Input: dimensioned drawing with shaded views. Units: mm. Origin: part minimum x, y, z. A direction names the side the tool comes from. Coordinates: 2 decimals unless noted, no trailing zeros. Write each loop counter-clockwise with the first axis right and the second up, starting at its lowest first coordinate (ties: lowest second). Pieces come first, ordered by that corner, then holes. Notation, with made-up numbers: (74, 83) -> (82, 83) arc R24 ccw to (82, 122) -> close; hole circle Ø3 at (-26.5, 32.25). An arc over 180 degrees is marked (long way). One line per item, written item: value. Start each with the question number.
1. First-contact query: P1, Ø1.5, axis at y = 4.5, z = 11.5, coming from the -X side; P2, Ø2, axis at x = 3.5, y = 7.5, coming from the +Z side; P3, Ø0.8, axis at x = 3.5, z = 18.5, coming from the -Y side; P4, Ø1, axis at y = 5.5, z = 17, coming from the +X side. Flat tips, straight axial feed; report the tip coordinate or a pass-through.
2. Section query A-A, the plane x = 4.25. Output: boundary loops of the cut face in (y, z).
3. Section query D-D, the plane y = 4.25. Output: boundary loops of the cut face in (x, z) (1 decimal).
4. Mould query, pull axis Z, two halves, no side actions, for the marked faces 1, 2, 3 and 4. Classes: released by +Z, released by -Z, zero draft, split by the parting line, or undercut.
5. Access query for the marked faces 5 and 6. Directions: +Z, -Z, +X, -X, +Y, -Y. A direction counts if a zero-diameter tool reaches every point of the face in a straight line with its end or side. Return the directions, or none.
6. Section query C-C, the plane z = 11.5. Output: boundary loops of the cut face in (x, y) (1 decimal), and give its area (3 significant figures).
7. Line query: line 1 (Z direction, x = 0.9, y = 4) (1 decimal); line 2 (Y direction, x = 3.75, z = 8.5); line 3 (Z direction, x = 2.5, y = 6.75). Output: solid intervals per line, ascending.
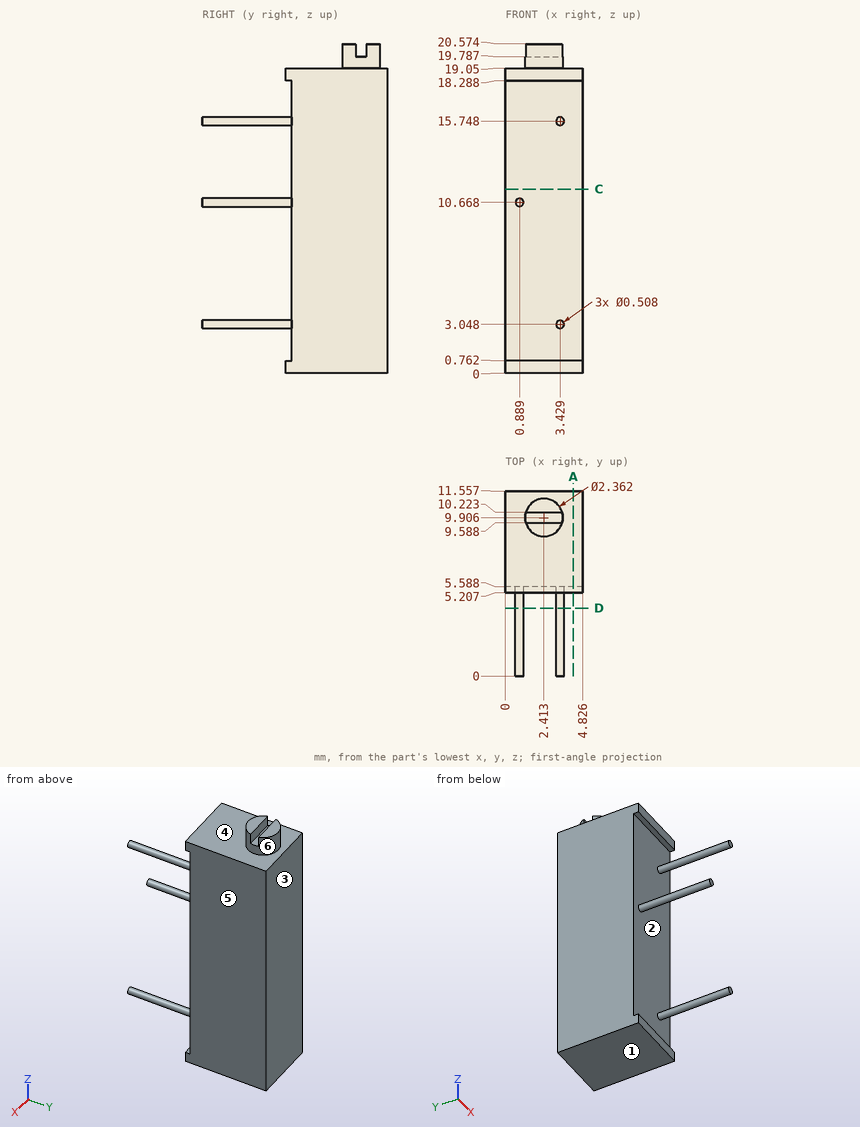
Computed values:
1. P1: stops at x = 0.65
1. P2: stops at z = 19.05
1. P3: stops at y = 5.21
1. P4: stops at x = 4.83
2. outline: (5.21, 0) -> (11.56, 0) -> (11.56, 19.05) -> (5.21, 19.05) -> (5.21, 18.29) -> (5.59, 18.29) -> (5.59, 0.76) -> (5.21, 0.76) -> close
3. outline: circle Ø0.5 at (0.9, 10.7); circle Ø0.5 at (3.4, 3); circle Ø0.5 at (3.4, 15.7)
4. face 1: released by -Z
4. face 2: undercut
4. face 3: zero draft
4. face 4: released by +Z
5. face 5: +Z, -Z, +X, +Y, -Y
5. face 6: +Z
6. outline: (0, 5.6) -> (4.8, 5.6) -> (4.8, 11.6) -> (0, 11.6) -> close
6. area: 28.8 mm²
7. line 1: z = 10.4 to 10.9
7. line 2: y = 5.59 to 11.56
7. line 3: z = 0 to 19.05
